Geometry: final body of the model. Coordinates: model frame, mm. Face numbers are marked on the shaded views. A direction names the side the tool comes from. Round coordinates to 2 decimals unless told otherwise and drop trailing zeros. Order: outer loops, then holes, each group sorted by start corner. A loop starts at its lowest first (then second) coordinate and runs counter-clockwise, first axis right, second up. Notation, with made-up numbers: M 5.25,52 L 56.25,52 A22 ccw 56.25,72 Z; hole C 46.5,29 d10. An arc over 180 degrees is marked long. Put each result on its own line as item: value. Start each with the question number.
1) Section A-A, the plane y = 0. Return loops of the section in (x, z).
2) Draft query along X for the marked faces 1 and 2. Return one class per face: pulls with the +X half, pulls with the -X half, needs draft (parallel to the pull), parting line crosses it, or undercut.
3) Access query for the marked faces 3 and 4. Directions: +Z, -Z, +X, -X, +Y, -Y. A direction counts if a zero-diameter tool reaches every point of the face in a straight line with its end or side. Return the directions, or none.
4) Section B-B, the plane x = -19.5. Return loops of the section in (y, z), then the cut area to 3 significant figures.
5) Material intervals for probe 1 along Y at (x, z) = (-14.5, 1.65); probe 2 along X at (y, z) = (7.75, 2.95); probe 3 along X at (y, z) = (-7.5, 1.95), sorted ascending. Write a range as [from, to].
6) First-contact query: P1, Ø5, axis at x = 16.97, y = 0, coming from the -Z side. Flat tip, straight axial feed; report the tip coordinate or a pass-through.
7) Section D-D, the plane z = 1.1. Return loops of the section in (x, y) (3 decimals).
8) Section C-C, the plane y = -6.75. Return loops of the section in (x, z).
from build123d import *

# Parameters (mm, degrees)
SKETCH1_W           = 74
SKETCH1_H           = 20
SKETCH1_R           = 2.125
SKETCH1_R_2         = 1.5
BOSS_EXTRUDE1_DEPTH = 4


with BuildPart() as part:
    # Sketch1 → Boss-Extrude1 (new body)
    with BuildSketch(Plane.XY):
        Rectangle(SKETCH1_W, SKETCH1_H)
        with Locations((32.221854305, 0)):
            Circle(SKETCH1_R, mode=Mode.SUBTRACT)
        with Locations((16.971854305, 0)):
            Circle(SKETCH1_R, mode=Mode.SUBTRACT)
        with Locations((-34.559305938, -7.559305938)):
            Circle(SKETCH1_R_2, mode=Mode.SUBTRACT)
        with Locations(Location((-34.559305938, 7.559305938, 0), (0, 0, 180))):
            Circle(SKETCH1_R_2, mode=Mode.SUBTRACT)
        with BuildLine():
            Line((-25.25, 4.75), (-5.75, 4.75))
            ThreePointArc((-5.75, 4.75), (-1, 0), (-5.75, -4.75))
            Line((-5.75, -4.75), (-25.25, -4.75))
            ThreePointArc((-25.25, -4.75), (-30, 0), (-25.25, 4.75))
        make_face(mode=Mode.SUBTRACT)
    extrude(amount=BOSS_EXTRUDE1_DEPTH)


solid = part.part
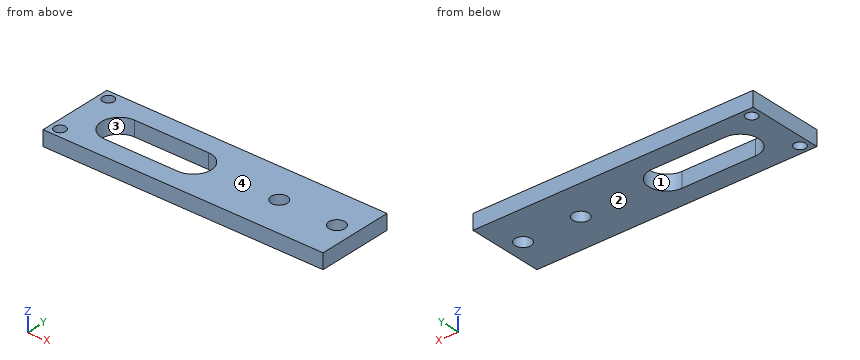
Result sheet:
1. outline: M -37,0 L -30,0 L -30,4 L -37,4 Z; M -1,0 L 14.85,0 L 14.85,4 L -1,4 Z; M 19.1,0 L 30.1,0 L 30.1,4 L 19.1,4 Z; M 34.35,0 L 37,0 L 37,4 L 34.35,4 Z
2. face 1: undercut
2. face 2: needs draft
3. face 3: +Z, -Z
3. face 4: +Z, +X, -X, +Y, -Y
4. outline: M -10,0 L -4.75,0 L -4.75,4 L -10,4 Z; M 4.75,0 L 10,0 L 10,4 L 4.75,4 Z
4. area: 42.0 mm2
5. probe 1: y = [-10, -4.75], [4.75, 10]
5. probe 2: x = [-37, -36.05], [-33.07, 37]
5. probe 3: x = [-37, -36.06], [-33.06, 37]
6. P1: stops at z = 0
7. outline: M -37,-10 L 37,-10 L 37,10 L -37,10 Z; hole C -34.559,-7.559 d3; hole C -34.559,7.559 d3; hole M -25.25,-4.75 L -5.75,-4.75 A4.75 ccw -5.75,4.75 L -25.25,4.75 A4.75 ccw Z; hole C 16.972,0 d4.25; hole C 32.222,0 d4.25
8. outline: M -37,0 L -35.82,0 L -35.82,4 L -37,4 Z; M -33.3,0 L 37,0 L 37,4 L -33.3,4 Z
